from build123d import *

# Parameters (mm, degrees)
EXTRUDE_1_DEPTH            = 217
FILLET_1_R                 = 20
SKETCH_4_W                 = 20
SKETCH_4_H                 = 8
CUT_EXTRUDE_3_DEPTH        = 10
PATTERN_LINEAR_1_COUNT     = 6
PATTERN_LINEAR_1_PITCH     = 24
PATTERN_LINEAR_1_COL_COUNT = 7
PATTERN_LINEAR_1_COL_PITCH = 24
FILLET_2_R                 = 6


with BuildPart() as part:
    # Эскиз1 → Бобышка-Вытянуть1 (new, symmetric)
    with BuildSketch(Plane.XY):
        Polygon((0, 0), (60, 0), (60, 6), (6, 6), (6, 60), (0, 60), align=None)
    extrude(amount=EXTRUDE_1_DEPTH, both=True)

    # Скругление1
    fillet_1_edges = [part.edges().sort_by_distance(p)[0] for p in [
        (60, 3, 217),
        (3, 60, 217),
        (3, 60, -217),
        (60, 3, -217),
    ]]
    fillet(fillet_1_edges, radius=FILLET_1_R)

    # Эскиз4 → Вырез-Вытянуть3 (cut)
    with BuildSketch(Plane(origin=(0, 0, 0), x_dir=(-1, 0, 0), z_dir=(0, -1, 0))):
        with Locations((-50, -12)):
            Rectangle(SKETCH_4_W, SKETCH_4_H)
    cut_extrude_3 = extrude(amount=-CUT_EXTRUDE_3_DEPTH, mode=Mode.SUBTRACT)

    # Линейный массив1: Вырез-Вытянуть3 ×6
    with Locations(*[(0, 0, i * PATTERN_LINEAR_1_PITCH) for i in range(1, PATTERN_LINEAR_1_COUNT)]):
        add(cut_extrude_3, mode=Mode.SUBTRACT)

    # Линейный массив1 col: Вырез-Вытянуть3 ×7
    with Locations(*[(0, 0, -i * PATTERN_LINEAR_1_COL_PITCH) for i in range(1, PATTERN_LINEAR_1_COL_COUNT)]):
        add(cut_extrude_3, mode=Mode.SUBTRACT)

    # Скругление2
    fillet_2_edges = [part.edges().sort_by_distance(p)[0] for p in [
        (6, 6, 0),
    ]]
    fillet(fillet_2_edges, radius=FILLET_2_R)


solid = part.part
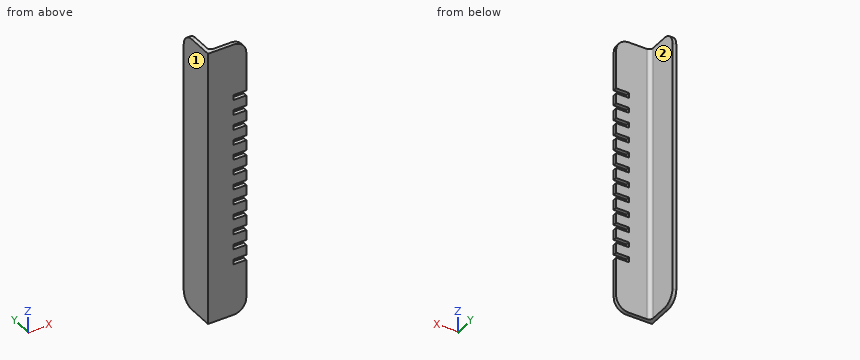
Read the model definition and answer for the solid it produces. Units are mm, in the model's axes. Face numbers are marked on the shaded views. A direction names the side the tool comes from. Coordinates: 2 decimals unless noted, no trailing zeros. Write each loop counter-clockwise with the first axis right and the second up, starting at its lowest first coordinate (ties: lowest second). Pieces come first, ordered by that corner, then holes. Notation, with made-up numbers: (75, -35.5) - (97, -35.5) arc R7 cw to (97, -23.5) - close; hole circle Ø6 at (14.5, 22.25). An arc over 180 degrees is marked (long way). One line per question, with ' | ' between items.
Q1. Consider L1, parallel to Y at x = 23, z = 110.5; L2, parallel to X at y = 5.5, z = -134.5. Determine where each line is inside the solid, lowest interval first. Write a range as [from, to].
Result set:
L1: [0, 6] | L2: [0, 40]
Q2. Find section B-B, the plane x = 28.5. Write down the section's boundary in (y, z), plus the area to 3 significant figures.
Result set:
outline: (0, -217) - (6, -217) - (6, 217) - (0, 217) - close | area: 2,600 mm^2
Q3. Find section A-A, the plane z = -12. Write down the section's boundary in (x, y), plus the area to 3 significant figures.
Result set:
outline: (0, 0) - (40, 0) - (40, 6) - (12, 6) arc R6 cw to (6, 12) - (6, 60) - (0, 60) - close | area: 572 mm^2
Q4. Find section D-D, the plane z = -99.5. Write down the section's boundary in (x, y).
Result set:
outline: (0, 0) - (60, 0) - (60, 6) - (12, 6) arc R6 cw to (6, 12) - (6, 60) - (0, 60) - close
Q5. Each of these flat-tipped pins is pushed along its axis until it touches: P1, Ø6.5, axis at y = 1.5, z = 12, coming from the +X side; P2, Ø3, axis at x = 48, y = 4, coming from the +Z side; P3, Ø1.8, axis at x = 54, y = 3, coming from the -Z side; P4, Ø10, axis at y = 6.5, z = 150, coming from the -X side. Where does it stop, or does it pass through?
Result set:
P1: x = 40 | P2: z = 215.91 | P3: z = -212.11 | P4: x = 0
Q6. For the marked faces 1 and 2, determine the directions among +Z, -Z, +X, -X, +Y, -Y from which every point of the face is accessible in a straight line to the end or side of a thin tool.
Result set:
face 1: +Z, -Z, -X, +Y, -Y | face 2: +Z, -Z, +X, +Y
